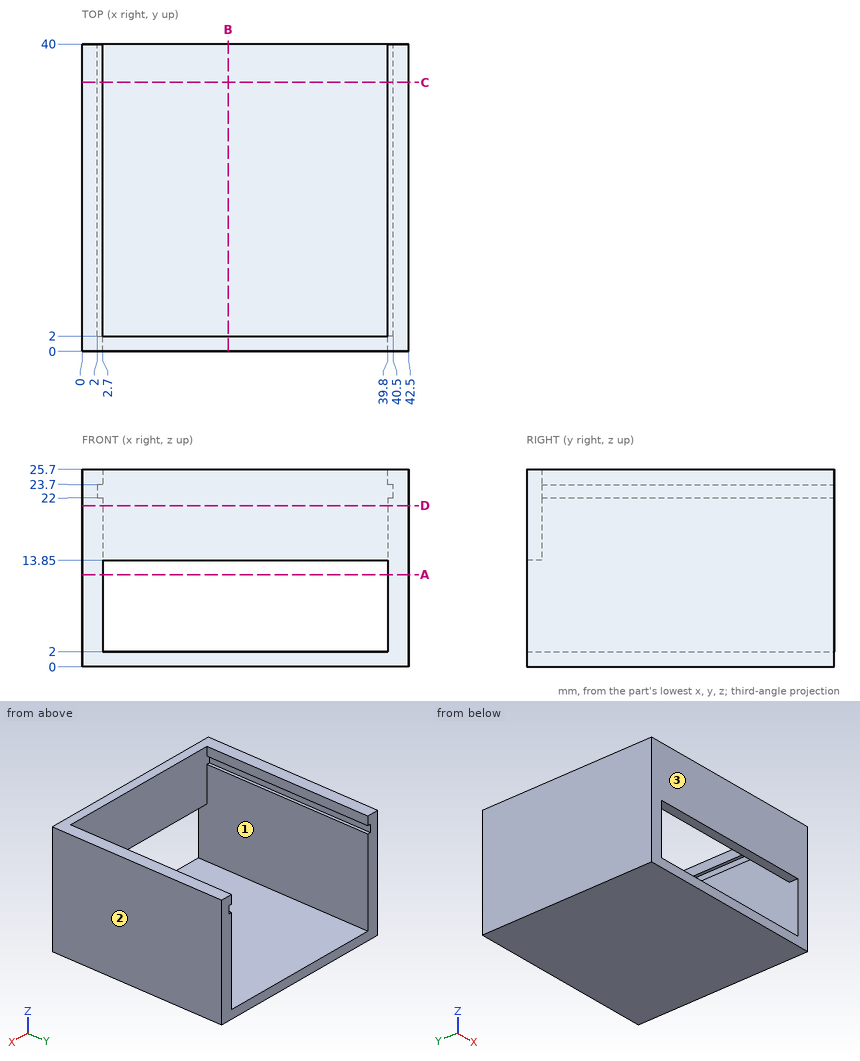
Drawing for the job (mm, zero at the part's lowest x, y, z). Give positions to 0.01 mm unless a question says otherwise; leave off trailing zeros. Loops run counter-clockwise (first coordinate to the right, second up) from the corner with the lowest first, then second, coordinate; pieces in that order, holes last.
(1) Band-saw the part on D-D (z = 21). Write the cut outline in (x, y).
Return value:
outline: (0, 0) - (42.5, 0) - (42.5, 40) - (39.8, 40) - (39.8, 2) - (2.7, 2) - (2.7, 40) - (0, 40) - close
(2) Band-saw the part on B-B (x = 19). Write the cut outline in (y, z), and give its area (3 significant figures).
Return value:
outline: (0, 0) - (40, 0) - (40, 2) - (0, 2) - close; (0, 13.85) - (2, 13.85) - (2, 25.7) - (0, 25.7) - close
area: 104 mm2
(3) Pin check, flat tips, straight feed: pin 1 (10 mm diameter, centred on x = 9.5, y = 31, fed in from +Z); pin 2 (1.5 mm diameter, centred on x = 31.5, z = 3.5, fed in from +Y); pin 3 (9.5 mm diameter, centred on x = 16.5, z = 20, fed in from +Y). Stop position of each tip, or through.
Return value:
pin 1: stops at z = 2
pin 2: passes through
pin 3: stops at y = 2
(4) Pull direction X, two halves, no side cores. Call the marked faces 1, 2 and 3: pulls with the +X half, pulls with the -X half, needs draft (parallel to the pull), parting line crosses it, or undercut.
Return value:
face 1: undercut
face 2: pulls with the +X half
face 3: needs draft
(5) Band-saw the part on C-C (y = 35). Write the cut outline in (x, z), and give its area (3 significant figures).
Return value:
outline: (0, 0) - (42.5, 0) - (42.5, 25.7) - (39.8, 25.7) - (39.8, 23.7) - (40.5, 23.7) - (40.5, 22) - (39.8, 22) - (39.8, 2) - (2.7, 2) - (2.7, 22) - (2, 22) - (2, 23.7) - (2.7, 23.7) - (2.7, 25.7) - (0, 25.7) - close
area: 211 mm2
(6) Band-saw the part on A-A (z = 12). Write the cut outline in (x, y), and give its area (3 significant figures).
Return value:
outline: (0, 0) - (2.7, 0) - (2.7, 40) - (0, 40) - close; (39.8, 0) - (42.5, 0) - (42.5, 40) - (39.8, 40) - close
area: 216 mm2
(7) Drill centre lines: line 1 along X through (y, z) = (9, 10.5); line 2 along Z through (x, y) = (28, 9); line 3 along Z through (x, y) = (40, 26.5). Where is each one in solid material? Low to high.
Return value:
line 1: x = 0 to 2.7, 39.8 to 42.5
line 2: z = 0 to 2
line 3: z = 0 to 22, 23.7 to 25.7
